Read the model definition and answer for the solid it produces. Units are mm, in the model's axes. A direction names the side the tool comes from. Coordinates: 2 decimals unless noted, no trailing zeros. Order: outer loops, then holes, each group sorted by start corner. A loop starts at its lowest first (then second) coordinate and runs counter-clockwise, first axis right, second up. Notation, with made-up numbers: M 37,44 L 82,44 A21 ccw 82,66 Z; hole C 82,32.25 d5. An arc over 180 degrees is marked long. Write each question's results on one line, items separated by ' | '.
```python
from build123d import *

# Parameters (mm, degrees)
SKETCH2_R                = 11.25
BOSS_EXTRUDE1_DEPTH      = 30
BOSS_EXTRUDE1_DEPTH_BACK = 50
BOSS_EXTRUDE2_REACH      = 76.743
SKETCH4_R                = 8.75
BOSS_EXTRUDE3_REACH      = 87.629
SKETCH11_R               = 6


with BuildPart() as part:
    # Sketch2 → Boss-Extrude1 (new body, two sides)
    with BuildSketch(Plane(origin=(0, 0, 0), x_dir=(1, 0, 0), z_dir=(0, 1, 0))) as boss_extrude1_sk:
        Circle(SKETCH2_R)
    extrude(amount=BOSS_EXTRUDE1_DEPTH)
    extrude(boss_extrude1_sk.sketch, amount=-BOSS_EXTRUDE1_DEPTH_BACK)

    # Sketch4 → Boss-Extrude2 (add, up to next)
    with BuildSketch(Plane(origin=(0, -25, 43.301270189), x_dir=(1, 0, 0), z_dir=(0, -0.5, 0.866025404)), mode=Mode.PRIVATE) as boss_extrude2_sk1:
        Circle(SKETCH4_R)
    boss_extrude2_tool1 = extrude(boss_extrude2_sk1.sketch, amount=-BOSS_EXTRUDE2_REACH, mode=Mode.PRIVATE) - part.part
    add(boss_extrude2_tool1.solids().sort_by_distance((0, -25, 43.30127))[0])

    # Sketch11 → Boss-Extrude3 (add, up to next)
    with BuildSketch(Plane(origin=(12.990381057, -15, -22.5), x_dir=(-0.901387819, -0.240192231, -0.360288346), z_dir=(0.433012702, -0.5, -0.75)), mode=Mode.PRIVATE) as boss_extrude3_sk1:
        Circle(SKETCH11_R)
    boss_extrude3_tool1 = extrude(boss_extrude3_sk1.sketch, amount=-BOSS_EXTRUDE3_REACH, mode=Mode.PRIVATE) - part.part
    add(boss_extrude3_tool1.solids().sort_by_distance((12.990381, -15, -22.5))[0])


solid = part.part
```
(1) Given pin 1 (10 mm diameter, centred on y = -31.5, z = 36.5, fed in from -X); pin 2 (1 mm diameter, centred on x = 0.5, y = 11.5, fed in from -Z); pin 3 (4 mm diameter, centred on y = -4, z = 19, fed in from +X), each flat-ended and moving along its own axis, determine where each tip first touches the part or whether it passes through.
Conclusion:
pin 1: x = -7.77 | pin 2: z = -11.25 | pin 3: x = 7.76
(2) The part is cut by section C-C, the plane y = 25. Write down the section's boundary in (x, z), then the cut area to 3 significant figures.
Conclusion:
outline: C 0,0 d22.5 | area: 398 mm²
(3) Straight lines are drawn through the part: line 1 (Z direction, x = 16.75, y = -14); line 2 (Z direction, x = -5.25, y = 9); line 3 (X direction, y = -14.5, z = 30.5). For each, find the intervals that lie inside material, in ascending order.
Conclusion:
line 1: -21 to -17.06 | line 2: -9.95 to 9.95 | line 3: -8.33 to 8.33
(4) For faces 1 (the cylindrical face through (-8.292, -9.44, -7.603)), 2 (the flat face through (13.066, -14.91, -22.516)), determine the directions among +Z, -Z, +X, -X, +Y, -Y from which every point of the face is accessible in a straight line to the end or side of a thin tool.
Conclusion:
face 1: none | face 2: -Z, +X, -Y
(5) The part is cut by section B-B, the plane x = -4. Write down the section's boundary in (y, z).
Conclusion:
outline: M -50,-10.51 L 30,-10.51 L 30,10.51 L 2.92,10.51 L -18.26,47.19 L -31.74,39.41 L -15.06,10.51 L -50,10.51 Z
(6) The part is cut by section D-D, the plane y = -18.5. Count the separate pieces of the cut face and the enclosed holes in it, then the cut area to 3 significant figures.
Conclusion:
separate pieces: 3 | enclosed holes: 0 | area: 888 mm²
(7) The part is cut by section A-A, the plane z = 0. Write down the section's boundary in (x, y).
Conclusion:
outline: M -11.25,-50 L 11.25,-50 L 11.25,30 L -11.25,30 Z
(8) The mould has two halves that part along Z. Classify faces 3 (the cylindrical face through (-1.14, -6.9, 29.3)), 4 (the flat face through (0, -50, 0)), 5 (the flat face through (-0.122, -24.894, 43.363)): pulls with the +Z half, pulls with the -Z half, needs draft (parallel to the pull), parting line crosses it, or undercut.
Conclusion:
face 3: undercut | face 4: needs draft | face 5: pulls with the +Z half
